from build123d import *

# Parameters (mm, degrees)
SKETCH1_W           = 10
SKETCH1_H           = 10
SKETCH1_W_2         = 8
SKETCH1_H_2         = 8
BOSS_EXTRUDE1_DEPTH = 340
SKETCH2_R           = 2.025
CUT_EXTRUDE1_DEPTH  = 341.183773863
SKETCH3_R           = 2.028
SKETCH3_R_2         = 2.025
CUT_EXTRUDE2_DEPTH  = 341.183773863
SKETCH4_W           = 10
SKETCH4_H           = 19
CUT_EXTRUDE3_DEPTH  = 341.183773863


with BuildPart() as part:
    # Sketch1 → Boss-Extrude1 (new body)
    with BuildSketch(Plane(origin=(0, 0, 0), x_dir=(1, 0, 0), z_dir=(0, 1, 0))):
        Rectangle(SKETCH1_W, SKETCH1_H)
        Rectangle(SKETCH1_W_2, SKETCH1_H_2, mode=Mode.SUBTRACT)
    extrude(amount=BOSS_EXTRUDE1_DEPTH)

    # Sketch2 → Cut-Extrude1 (cut, through all)
    with BuildSketch(Plane.XY.offset(5)):
        with Locations((0, 90)):
            Circle(SKETCH2_R)
        with Locations((0, 30)):
            Circle(SKETCH2_R)
        with Locations((0, 24)):
            Circle(SKETCH2_R)
    extrude(amount=-CUT_EXTRUDE1_DEPTH, mode=Mode.SUBTRACT)

    # Sketch3 → Cut-Extrude2 (cut, through all)
    with BuildSketch(Plane(origin=(5, 0, 0), x_dir=(0, 0, -1), z_dir=(1, 0, 0))):
        with Locations((0, 312)):
            Circle(SKETCH3_R)
        with Locations((0, 297)):
            Circle(SKETCH3_R_2)
        with Locations((0, 147)):
            Circle(SKETCH3_R_2)
        with Locations((0, 132)):
            Circle(SKETCH3_R_2)
    extrude(amount=-CUT_EXTRUDE2_DEPTH, mode=Mode.SUBTRACT)

    # Sketch4 → Cut-Extrude3 (cut, through all)
    with BuildSketch(Plane.XY.offset(5)):
        with Locations((0, 9.5)):
            Rectangle(SKETCH4_W, SKETCH4_H)
    extrude(amount=-CUT_EXTRUDE3_DEPTH, mode=Mode.SUBTRACT)


solid = part.part
Source: CAD feature listing. Evaluate the final solid. Frame: model axes, mm. A direction names the side the tool comes from. Round coordinates to 2 decimals unless told otherwise and drop trailing zeros. Order: outer loops, then holes, each group sorted by start corner. A loop starts at its lowest first (then second) coordinate and runs counter-clockwise, first axis right, second up. Notation, with made-up numbers: (-11.5, -12.5) -> (19.5, -12.5) arc R19 cw to (19.5, 22.5) -> close; hole circle Ø1 at (-33, 35). An arc over 180 degrees is marked (long way). Answer as CSV lines item,"result".
Item 1: Pull-direction query (X, two-part tool) for faces 3 (the face through (0, 177, -5)), 4 (the face through (0, 177, 4)), 5 (the face through (-4, 177, 0)), 6 (the face through (5, 177, 0)); classes: pulls with the +X half, pulls with the -X half, needs draft (parallel to the pull), parting line crosses it, or undercut.
A:
face 3,"needs draft"
face 4,"undercut"
face 5,"undercut"
face 6,"pulls with the +X half"
Item 2: Section A-A, the plane x = 0. Count the separate pieces of the cut face and the enclosed holes in it, plus the area to 3 significant figures.
A:
separate pieces,"8"
enclosed holes,"0"
area,"618 mm²"
Item 3: Section B-B, the plane y = 242. Return loops of the section in (x, z), plus the area to 3 significant figures.
A:
outline,"(-5, -5) -> (5, -5) -> (5, 5) -> (-5, 5) -> close; hole (-4, -4) -> (4, -4) -> (4, 4) -> (-4, 4) -> close"
area,"36.0 mm²"
Item 4: Pin query (flat end, axial travel): pin 1 Ø2.5 at (y, z) = (297, 0) entering from +X; pin 2 Ø5.5 at (x, y) = (0, 30) entering from +Z. Return the tip coordinate at first contact, or that it passes through.
A:
pin 1,"through"
pin 2,"z = 5"
Item 5: Line query: L1, parallel to Y at x = 0, z = -4.15 (3 decimals); L2, parallel to Y at x = 4.7, z = 0 (3 decimals); L3, parallel to Z at x = -4.5, y = 312. Output: solid intervals per line, ascending.
A:
L1,"19 to 21.975, 26.025 to 27.975, 32.025 to 87.975, 92.025 to 340"
L2,"19 to 129.975, 134.025 to 144.975, 149.025 to 294.975, 299.025 to 309.972, 314.028 to 340"
L3,"-5 to -2.03, 2.03 to 5"
Item 6: Reachability of faces 1 (the face through (4, 177, 0)), 2 (the face through (0, 177, 5)) from +Z, -Z, +X, -X, +Y, -Y: full face, straight path, thin tool, end or side. Return the list, or none.
A:
face 1,"+Y, -Y"
face 2,"+Z, +X, -X, +Y, -Y"
